Geometry check sheet. Reference: drawing and pictorial views, mm from the part's lowest x, y, z. Give positions to 0.01 mm unless a question says otherwise; leave off trailing zeros. Order: outer loops, then holes, each group sorted by start corner. A loop starts at its lowest first (then second) coordinate and runs counter-clockwise, first axis right, second up. Notation, with made-up numbers: (11, 37.5) -> (33, 37.5) arc R15 ccw to (33, 51.5) -> close; hole circle Ø9 at (75, 36). An arc over 180 degrees is marked (long way). Write each question's results on one line, items separated by ' | '.
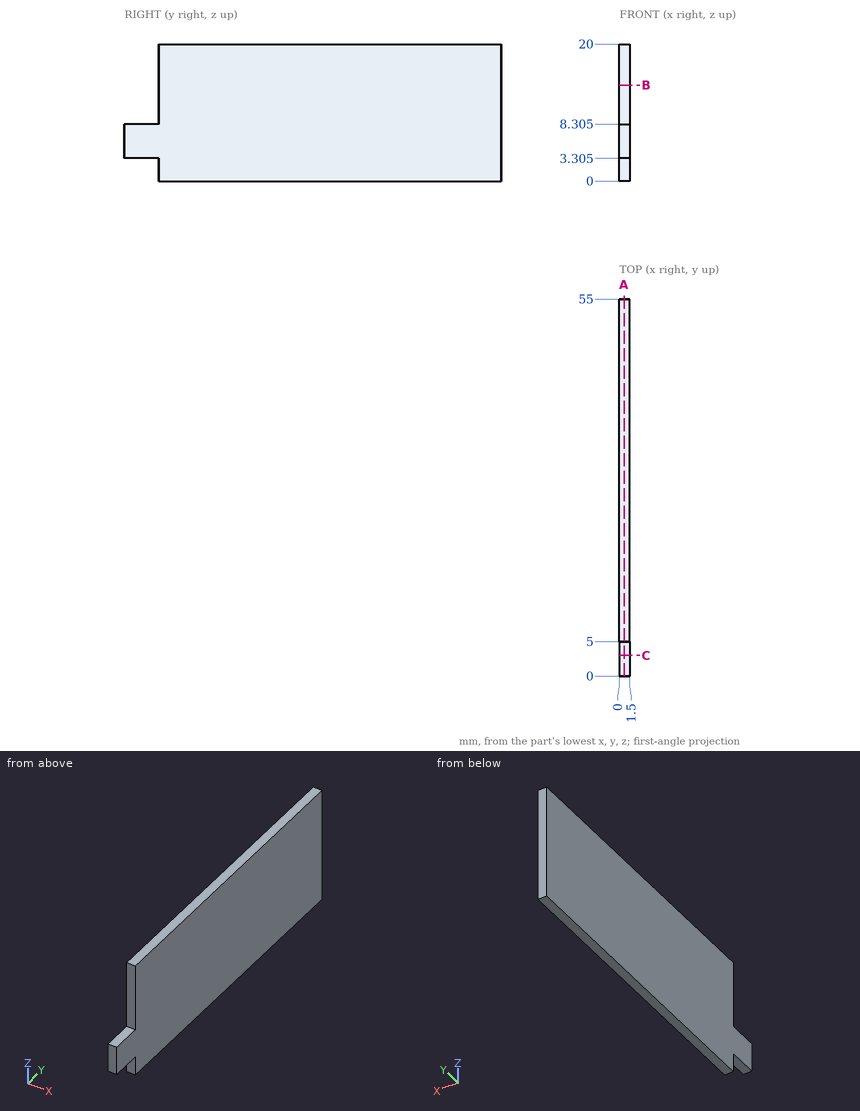
1. Section check B-B on z = 14. Record the cut outline in (x, y).
Verdict:
outline: (0, 5) -> (1.5, 5) -> (1.5, 55) -> (0, 55) -> close
2. Section check C-C on y = 3. Record the cut outline in (x, z) (1 decimal).
Verdict:
outline: (0, 3.3) -> (1.5, 3.3) -> (1.5, 8.3) -> (0, 8.3) -> close
3. Section check A-A on x = 0.7. Record the cut outline in (y, z) (1 decimal), then the cut area to 4 significant figures.
Verdict:
outline: (0, 3.3) -> (5, 3.3) -> (5, 0) -> (55, 0) -> (55, 20) -> (5, 20) -> (5, 8.3) -> (0, 8.3) -> close | area: 1,025 mm^2
4. Material ranges on probe 1 along Y at (x, z) = (0.2, 17.75); probe 2 along Z at (x, y) = (0.5, 3.5) (1 decimal), recorded low to high. Write a range as from..to.
Verdict:
probe 1: y = 5..55 | probe 2: z = 3.3..8.3
